Autodesk Inventor part; units mm, degrees
ref_plane "YZ Plane" through (0, 0, 0) normal (1, 0, 0) x (0, 1, 0)
ref_plane "XZ Plane" through (0, 0, 0) normal (0, 1, 0) x (-1, 0, 0)
ref_plane "XY Plane" through (0, 0, 0) normal (0, 0, 1) x (1, 0, 0)
sketch "Sketch1" plane through (0, 0, 0) normal (0, 1, 0) x (-1, 0, 0)
  circle A0 centre (0, 0) radius 7
  circle A1 centre (0, 0) radius 16
  circle A2 centre (8, 8) radius 2
  circle A3 centre (-8, 8) radius 2
  circle A4 centre (-8, -8) radius 2
  circle A5 centre (8, -8) radius 2
  dimension "d0" = 14
  dimension "d1" = 32
  dimension "d4" = 4
  dimension "d5" = 8
  dimension "d6" = 8
  dimension "d9" = 360
extrude "Extrusion1" add sketch "Sketch1" along normal blind 24
properties part number "MotorPulleySpacer"
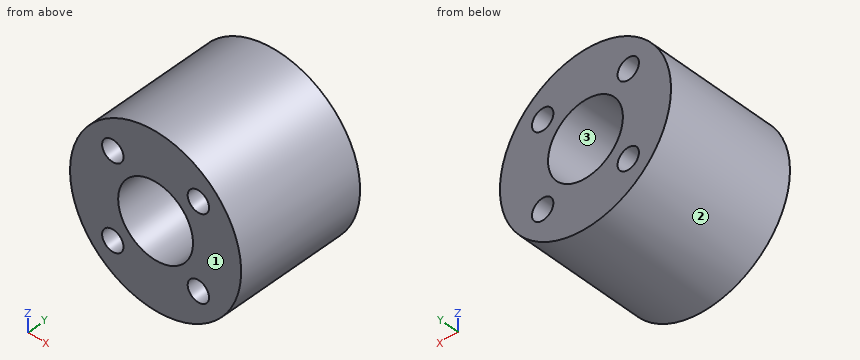
Verification items for the finished model (mm, model axes). Face numbers are marked on the shaded views. Round coordinates to 2 decimals unless told otherwise and drop trailing zeros. Loops run counter-clockwise (first coordinate to the right, second up) from the corner with the lowest first, then second, coordinate; pieces in that order, holes last. Notation, with made-up numbers: (32.25, 73) - (84.25, 73) arc R13 ccw to (84.25, 82) - close; hole circle Ø2 at (39, 75.5). An arc over 180 degrees is marked (long way). Use one line per item in the form item = value.
1. Draft check along Z on the marked faces 1, 2 and 3. Enter one of: pulls with the +Z half, pulls with the -Z half, needs draft (parallel to the pull), parting line crosses it, or undercut.
A:
face_1 = needs draft
face_2 = parting line crosses it
face_3 = undercut
2. Section check A-A on x = 0. Record the cut outline in (y, z).
A:
outline = (0, -16) - (24, -16) - (24, -7) - (0, -7) - close; (0, 7) - (24, 7) - (24, 16) - (0, 16) - close
3. Section check D-D on z = 8. Record the cut outline in (x, y), and give its area (3 significant figures).
A:
outline = (-13.86, 0) - (-10, 0) - (-10, 24) - (-13.86, 24) - close; (-6, 0) - (6, 0) - (6, 24) - (-6, 24) - close; (10, 0) - (13.86, 0) - (13.86, 24) - (10, 24) - close
area = 473 mm²
4. Scan lines: probe 1 along X at (y, z) = (18.25, -9.5); probe 2 along Z at (x, y) = (-9, 22.25); probe 3 along Z at (x, y) = (-7.5, 11.75). Record each from-to range of solid material in increasing order.
A:
probe_1 = -12.87 to -9.32, -6.68 to 6.68, 9.32 to 12.87
probe_2 = -13.23 to -9.73, -6.27 to 6.27, 9.73 to 13.23
probe_3 = -14.13 to -9.94, -6.06 to 6.06, 9.94 to 14.13
5. Section check B-B on z = 0. Record the cut outline in (x, y), and give its area (3 significant figures).
A:
outline = (-16, 0) - (-7, 0) - (-7, 24) - (-16, 24) - close; (7, 0) - (16, 0) - (16, 24) - (7, 24) - close
area = 432 mm²
6. Gauge pin test, flat ends, axial feed: pin 1 Ø12 at (y, z) = (6.5, -4.5) entering from +X; pin 2 Ø3 at (x, z) = (-8, -8) entering from -Y; pin 3 Ø1.5 at (x, y) = (5.5, 7) entering from +Z; pin 4 Ø5 at (y, z) = (20.5, 8) entering from -X (3 decimals). Record the tip position at first contact, or that the pin passes through.
A:
pin_1 = 16
pin_2 = through
pin_3 = 15.28
pin_4 = -15.025
7. Section check C-C on y = 20.5. Record the cut outline in (x, z), and give its area (3 significant figures).
A:
outline = circle Ø32 at (0, 0); hole circle Ø4 at (-8, -8); hole circle Ø4 at (-8, 8); hole circle Ø14 at (0, 0); hole circle Ø4 at (8, -8); hole circle Ø4 at (8, 8)
area = 600 mm²
